Model file for the job. Use its own axes, mm. Face numbers are marked on the shaded views. A direction names the side the tool comes from. Round coordinates to 2 decimals unless told otherwise and drop trailing zeros. Loops run counter-clockwise (first coordinate to the right, second up) from the corner with the lowest first, then second, coordinate; pieces in that order, holes last. Notation, with made-up numbers: M 10.5,76 L 53.5,76 A22 cw 53.5,96 Z; hole C 61,60 d11. An arc over 180 degrees is marked long. Use a Markdown table: item, result. Add a question column.
Item 1: Saw through at B-B on z = 8.75. Write the cut outline in (x, y), then the cut area to 3 significant figures.
Item 2: Two-plate mould, pull along Z, no slides. Class the marked faces 5, 6 and 7: +Z half, -Z half, draft (parallel to the pull), parting line (faces both ways), or undercut.
Item 3: Wall check: L1, parallel to Y at x = -23.75, z = 21.25; L2, parallel to Y at x = -23.5, z = 21; L3, parallel to Z at x = -21.25, y = 8.25. Give the ranges that are in metal, low to high. Write a range as from..to.
Item 4: Tool access for the marked faces 1, 2, 3 and 4: list every direction of +Z, -Z, +X, -X, +Y, -Y with a clear straight run to the whole face (end or side of a thin tool).
Item 5: Saw through at A-A on z = 13.5. Write the cut outline in (x, y).
Item 6: Saw through at C-C on z = 16.5. Write the cut outline in (x, y), then the cut area to 3 significant figures.
Item 7: Pin check, flat tips, straight feed: P1, Ø1.2, axis at x = -26, y = 2, coming from the +Z side; P2, Ø4, axis at x = -24.5, y = 5.5, coming from the -Z side. Stop position of each tip, or through.
```python
from build123d import *

# Parameters (mm, degrees)
SPUR_START                  = -26.948632746
SPUR_GEAR_ISO_OUTLINE_R     = 2.5
SPUR_GEAR_ISO_DEPTH         = 6
SPUR_START_2                = -28.948683546
SPUR_GEAR_ISO_2_OUTLINE_R   = 5
SPUR_GEAR_ISO_2_OUTLINE_R_2 = 2.5
SPUR_GEAR_ISO_2_DEPTH       = 2.0000508
BOSS_EXTRUDE1_DEPTH         = 8.0000508


# Read off the part's stored shape, not the designer's step: spur gear_iso
with BuildPart() as part:
    # spur gear_iso outline → spur gear_iso (new body)
    with BuildSketch(Plane.YZ.offset(SPUR_START)):
        with BuildLine():
            ThreePointArc((9.06624461, 20.039929061), (8.809867644, 20.262580741), (8.54607915, 20.476399706))
            ThreePointArc((8.54607915, 20.476399706), (7.532383697, 19.882145035), (6.764050297, 18.993111362))
            ThreePointArc((6.764050297, 18.993111362), (6.256491547, 19.312967164), (5.725708923, 19.592598034))
            ThreePointArc((5.725708923, 19.592598034), (6.111467968, 20.702511114), (6.119259883, 21.877524463))
            ThreePointArc((6.119259883, 21.877524463), (5.802192981, 21.999062518), (5.481182486, 22.109765643))
            ThreePointArc((5.481182486, 22.109765643), (4.731867417, 21.20464465), (4.313937615, 20.106440768))
            ThreePointArc((4.313937615, 20.106440768), (3.727591276, 20.233411588), (3.13317937, 20.314640304))
            ThreePointArc((3.13317937, 20.314640304), (3.116061668, 21.489554798), (2.721505439, 22.596371164))
            ThreePointArc((2.721505439, 22.596371164), (2.381991548, 22.60213631), (2.042477656, 22.596371164))
            ThreePointArc((2.042477656, 22.596371164), (1.647921427, 21.489554798), (1.630803724, 20.314640304))
            ThreePointArc((1.630803724, 20.314640304), (1.036391818, 20.233411588), (0.45004548, 20.106440768))
            ThreePointArc((0.45004548, 20.106440768), (0.032115678, 21.20464465), (-0.717199391, 22.109765643))
            ThreePointArc((-0.717199391, 22.109765643), (-1.038209886, 21.999062518), (-1.355276788, 21.877524463))
            ThreePointArc((-1.355276788, 21.877524463), (-1.347484873, 20.702511114), (-0.961725828, 19.592598034))
            ThreePointArc((-0.961725828, 19.592598034), (-1.492508453, 19.312967164), (-2.000067202, 18.993111362))
            ThreePointArc((-2.000067202, 18.993111362), (-2.768400602, 19.882145035), (-3.782096055, 20.476399706))
            ThreePointArc((-3.782096055, 20.476399706), (-4.045884549, 20.262580741), (-4.302261515, 20.039929061))
            ThreePointArc((-4.302261515, 20.039929061), (-3.893061276, 18.938442679), (-3.150953717, 18.027402912))
            ThreePointArc((-3.150953717, 18.027402912), (-3.554086842, 17.583097498), (-3.921638927, 17.108936045))
            ThreePointArc((-3.921638927, 17.108936045), (-4.947703578, 17.681568927), (-6.103512782, 17.893281392))
            ThreePointArc((-6.103512782, 17.893281392), (-6.27826249, 17.60213631), (-6.443026673, 17.305226082))
            ThreePointArc((-6.443026673, 17.305226082), (-5.681773697, 16.410122182), (-4.672826749, 15.807840569))
            ThreePointArc((-4.672826749, 15.807840569), (-4.899686571, 15.252450401), (-5.082899784, 14.681174166))
            ThreePointArc((-5.082899784, 14.681174166), (-6.242937146, 14.868338281), (-7.401452454, 14.671972892))
            ThreePointArc((-7.401452454, 14.671972892), (-7.466085983, 14.338618087), (-7.519364391, 14.003261067))
            ThreePointArc((-7.519364391, 14.003261067), (-6.497877023, 13.422502389), (-5.343784577, 13.201622982))
            ThreePointArc((-5.343784577, 13.201622982), (-5.367008453, 12.60213631), (-5.343784577, 12.002649638))
            ThreePointArc((-5.343784577, 12.002649638), (-6.497877023, 11.781770232), (-7.519364391, 11.201011553))
            ThreePointArc((-7.519364391, 11.201011553), (-7.466085983, 10.865654533), (-7.401452454, 10.532299728))
            ThreePointArc((-7.401452454, 10.532299728), (-6.242937146, 10.335934339), (-5.082899784, 10.523098454))
            ThreePointArc((-5.082899784, 10.523098454), (-4.899686571, 9.951822219), (-4.672826749, 9.396432051))
            ThreePointArc((-4.672826749, 9.396432051), (-5.681773698, 8.794150439), (-6.443026673, 7.899046538))
            ThreePointArc((-6.443026673, 7.899046538), (-6.27826249, 7.60213631), (-6.103512782, 7.310991228))
            ThreePointArc((-6.103512782, 7.310991228), (-4.947703577, 7.522703693), (-3.921638927, 8.095336576))
            ThreePointArc((-3.921638927, 8.095336576), (-3.554086842, 7.621175123), (-3.150953717, 7.176869708))
            ThreePointArc((-3.150953717, 7.176869708), (-3.893061276, 6.265829942), (-4.302261515, 5.16434356))
            ThreePointArc((-4.302261515, 5.16434356), (-4.045884549, 4.941691879), (-3.782096055, 4.727872914))
            ThreePointArc((-3.782096055, 4.727872914), (-2.768400602, 5.322127585), (-2.000067202, 6.211161258))
            ThreePointArc((-2.000067202, 6.211161258), (-1.492508453, 5.891305456), (-0.961725828, 5.611674586))
            ThreePointArc((-0.961725828, 5.611674586), (-1.347484873, 4.501761506), (-1.355276788, 3.326748157))
            ThreePointArc((-1.355276788, 3.326748157), (-1.038209886, 3.205210102), (-0.717199391, 3.094506978))
            ThreePointArc((-0.717199391, 3.094506978), (0.032115678, 3.999627971), (0.45004548, 5.097831853))
            ThreePointArc((0.45004548, 5.097831853), (1.036391818, 4.970861032), (1.630803724, 4.889632316))
            ThreePointArc((1.630803724, 4.889632316), (1.647921427, 3.714717822), (2.042477656, 2.607901456))
            ThreePointArc((2.042477656, 2.607901456), (2.381991548, 2.60213631), (2.721505439, 2.607901456))
            ThreePointArc((2.721505439, 2.607901456), (3.116061668, 3.714717822), (3.13317937, 4.889632316))
            ThreePointArc((3.13317937, 4.889632316), (3.727591276, 4.970861032), (4.313937615, 5.097831853))
            ThreePointArc((4.313937615, 5.097831853), (4.731867417, 3.999627971), (5.481182486, 3.094506978))
            ThreePointArc((5.481182486, 3.094506978), (5.802192981, 3.205210102), (6.119259883, 3.326748157))
            ThreePointArc((6.119259883, 3.326748157), (6.111467968, 4.501761506), (5.725708923, 5.611674586))
            ThreePointArc((5.725708923, 5.611674586), (6.256491547, 5.891305456), (6.764050297, 6.211161258))
            ThreePointArc((6.764050297, 6.211161258), (7.532383697, 5.322127585), (8.54607915, 4.727872914))
            ThreePointArc((8.54607915, 4.727872914), (8.809867644, 4.941691879), (9.06624461, 5.16434356))
            ThreePointArc((9.06624461, 5.16434356), (8.657044371, 6.265829942), (7.914936812, 7.176869708))
            ThreePointArc((7.914936812, 7.176869708), (8.318069937, 7.621175123), (8.685622021, 8.095336576))
            ThreePointArc((8.685622021, 8.095336576), (9.711686672, 7.522703693), (10.867495877, 7.310991228))
            ThreePointArc((10.867495877, 7.310991228), (11.042245585, 7.60213631), (11.207009768, 7.899046538))
            ThreePointArc((11.207009768, 7.899046538), (10.445756793, 8.794150439), (9.436809844, 9.396432051))
            ThreePointArc((9.436809844, 9.396432051), (9.663669666, 9.951822219), (9.846882879, 10.523098454))
            ThreePointArc((9.846882879, 10.523098454), (11.006920241, 10.335934339), (12.165435549, 10.532299728))
            ThreePointArc((12.165435549, 10.532299728), (12.230069078, 10.865654533), (12.283347486, 11.201011553))
            ThreePointArc((12.283347486, 11.201011553), (11.261860118, 11.781770232), (10.107767672, 12.002649638))
            ThreePointArc((10.107767672, 12.002649638), (10.130991547, 12.60213631), (10.107767672, 13.201622982))
            ThreePointArc((10.107767672, 13.201622982), (11.261860118, 13.422502389), (12.283347486, 14.003261067))
            ThreePointArc((12.283347486, 14.003261067), (12.230069078, 14.338618087), (12.165435549, 14.671972892))
            ThreePointArc((12.165435549, 14.671972892), (11.006920241, 14.868338281), (9.846882879, 14.681174166))
            ThreePointArc((9.846882879, 14.681174166), (9.663669666, 15.252450401), (9.436809844, 15.807840569))
            ThreePointArc((9.436809844, 15.807840569), (10.445756792, 16.410122182), (11.207009768, 17.305226082))
            ThreePointArc((11.207009768, 17.305226082), (11.042245585, 17.60213631), (10.867495877, 17.893281392))
            ThreePointArc((10.867495877, 17.893281392), (9.711686672, 17.681568927), (8.685622021, 17.108936045))
            ThreePointArc((8.685622021, 17.108936045), (8.318069937, 17.583097498), (7.914936812, 18.027402912))
            ThreePointArc((7.914936812, 18.027402912), (8.657044371, 18.938442679), (9.06624461, 20.039929061))
        make_face()
        with Locations((2.381991547, 12.60213631)):
            Circle(SPUR_GEAR_ISO_OUTLINE_R, mode=Mode.SUBTRACT)
    extrude(amount=SPUR_GEAR_ISO_DEPTH)

    # spur gear_iso 2 outline → spur gear_iso 2 (add)
    with BuildSketch(Plane.YZ.offset(SPUR_START_2)):
        with Locations((2.381991547, 12.60213631)):
            Circle(SPUR_GEAR_ISO_2_OUTLINE_R)
        with Locations((2.381991547, 12.60213631)):
            Circle(SPUR_GEAR_ISO_2_OUTLINE_R_2, mode=Mode.SUBTRACT)
    extrude(amount=SPUR_GEAR_ISO_2_DEPTH)

    # Sketch1 → Boss-Extrude1 (add)
    with BuildSketch(Plane.ZY.offset(28.948683546)):
        with BuildLine():
            Line((11.10213631, 0.381991547), (11.10213631, 4.381991547))
            ThreePointArc((11.10213631, 4.381991547), (10.10213631, 2.381991547), (11.10213631, 0.381991547))
        make_face()
        with BuildLine():
            ThreePointArc((15.10213631, 2.381991547), (14.838204288, 3.500025536), (14.10213631, 4.381991547))
            Line((14.10213631, 4.381991547), (14.10213631, 0.381991547))
            ThreePointArc((14.10213631, 0.381991547), (14.838204288, 1.263957559), (15.10213631, 2.381991547))
        make_face()
    extrude(amount=-BOSS_EXTRUDE1_DEPTH)


solid = part.part
```
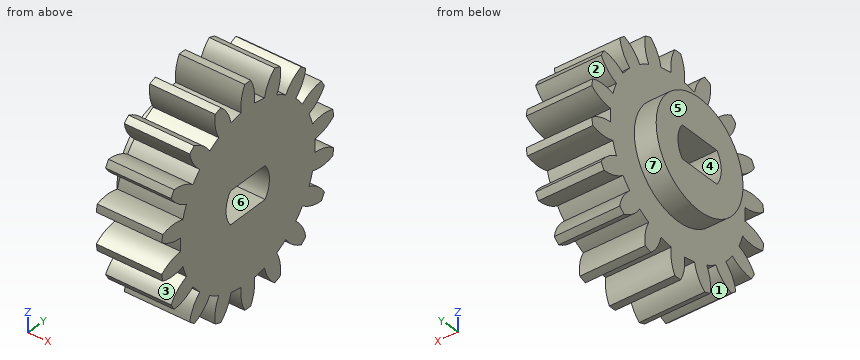
Entries:
| question | item | result |
|---|---|---|
| 1 | outline | M -28.95,-0.81 L -26.95,-0.81 L -26.95,-5.73 L -20.95,-5.73 L -20.95,10.5 L -26.95,10.5 L -26.95,5.57 L -28.95,5.57 Z |
| 1 | area | 110 mm2 |
| 2 | face 5 | draft |
| 2 | face 6 | undercut |
| 2 | face 7 | parting line |
| 3 | L1 | -1.4..0.01, 1.61..3.15, 4.76..6.16 |
| 3 | L2 | -1.39..0.14, 1.59..3.17, 4.62..6.15 |
| 3 | L3 | 4.86..6.84, 7.54..17.66, 18.37..20.35 |
| 4 | face 1 | -Z, +X, -X |
| 4 | face 2 | +X, -X, +Y |
| 4 | face 3 | +X, -X, -Y |
| 4 | face 4 | +X, -X |
| 5 | outline | M -28.95,-2.54 L -26.95,-2.54 L -26.95,-6.69 L -20.95,-6.69 L -20.95,0.05 L -28.95,0.05 Z; M -28.95,4.72 L -20.95,4.72 L -20.95,11.45 L -26.95,11.45 L -26.95,7.3 L -28.95,7.3 Z |
| 6 | outline | M -28.95,-0.75 L -26.95,-0.75 L -26.95,-5.78 L -20.95,-5.78 L -20.95,10.55 L -26.95,10.55 L -26.95,5.51 L -28.95,5.51 Z |
| 6 | area | 111 mm2 |
| 7 | P1 | z = 22.6 |
| 7 | P2 | z = 3.09 |
